Autodesk Inventor part; units mm, degrees
ref_plane "YZ Plane" through (0, 0, 0) normal (1, 0, 0) x (0, 1, 0)
ref_plane "XZ Plane" through (0, 0, 0) normal (0, 1, 0) x (-1, 0, 0)
ref_plane "XY Plane" through (0, 0, 0) normal (0, 0, 1) x (1, 0, 0)
sketch "Sketch1" plane through (0, 0, 0) normal (0, 1, 0) x (-1, 0, 0)
  circle A0 centre (0, 0) radius 1.5
  dimension "d1" = 3
extrude "Extrusion1" add sketch "Sketch1" along normal blind 6
sketch "Sketch2" plane through (0, 6, 0) normal (0, 1, 0) x (1, 0, 0)
  circle A0 centre (0, 0) radius 2.75
  dimension "d4" = 5.5
extrude "Extrusion2" add sketch "Sketch2" along normal blind 3
sketch "Sketch3" plane through (0, 9, 0) normal (0, 1, 0) x (1, 0, 0)
  line L0 (1.5, 0) -> (0.75, -1.299)
  line L1 (0.75, -1.299) -> (-0.75, -1.299)
  line L2 (-0.75, -1.299) -> (-1.5, 0)
  line L3 (-1.5, 0) -> (-0.75, 1.299)
  line L4 (-0.75, 1.299) -> (0.75, 1.299)
  line L5 (0.75, 1.299) -> (1.5, 0)
  point P0 (0, 0)
  point P1 (0, 0)
  dimension "d7" = 1.5
extrude "Extrusion3" cut sketch "Sketch3" against normal blind 2
thread "Thread1"
fillet "Fillet1" radius 0.3 2 edges at (-2.75, 6, 0) (-2.75, 9, 0)
chamfer "Chamfer1" distance 0.05 angle 45 1 edges at (1.5, 0, 0)
chamfer "Chamfer2" distance 0.05 angle 45 1 edges at (1.5, 6, 0)
fillet "Fillet2" radius 0.05 12 edges at (0, 9, -1.299) (1.125, 9, -0.6495) (1.125, 9, 0.6495) (0, 9, 1.299) (-1.125, 9, 0.6495) (-1.125, 9, -0.6495) (0, 7, -1.299) (1.125, 7, -0.6495) (1.125, 7, 0.6495) (-1.125, 7, -0.6495) (-1.125, 7, 0.6495) (0, 7, 1.299)
sketch "Sketch4" plane through (0, 0, 0) normal (0, -1, 0) x (1, 0, 0)
  circle A0 centre (0, 0) radius 1.425
  dimension "d21" = 2.85
extrude "Extrusion4" cut sketch "Sketch4" against normal blind 0.1
chamfer "Chamfer3" distance 0.05 angle 45 1 edges at (-1.425, 0.1, 0)
properties part number "L Bolt M3 x 6 Stainless Steel"
Build history of the part. All positions in model axes, mm. A direction names the side the tool comes from. Round coordinates to 2 decimals unless told otherwise and drop trailing zeros. Write each loop counter-clockwise with the first axis right and the second up, starting at its lowest first coordinate (ties: lowest second). Pieces come first, ordered by that corner, then holes. Notation, with made-up numbers: (-7, -19.75) - (44, -19.75) arc R22 ccw to (44, -1.75) - close; hole circle Ø10 at (82, -15.75). An arc over 180 degrees is marked (long way). Write each question's results on one line, items separated by ' | '. Start each with the question number.
Item 1: Which spindle directions (+Z, -Z, +X, -X, +Y, -Y) get a long thin tool onto all of the face, cutting with end or side? Do faces 1 (the face through (0, 6, 2)), 2 (the face through (0, 8, -1.299)), 3 (the face through (-0.596, 7.483, -2.685)). Say none if no direction does.
Item 2: Saw through at B-B (y = 1.5). Write the cut outline in (x, z), and give its area (3 significant figures).
Item 3: Mould opens along Z. For faces 4 (the face through (0, 7, 0)), 5 (the face through (-1.12, 8.01, 0.66)), 6 (the face through (1.5, 2.96, -0.07)), 7 (the face through (1.1, 9, 1.1)) say: pulls with the +Z half, pulls with the -Z half, needs draft (parallel to the pull), parting line crosses it, or undercut.
Item 4: Wall check: L1, parallel to Y at x = -0.4, z = -0.65; L2, parallel to Z at x = -1.3, y = 2.75; L3, parallel to Y at x = -1.9, z = -0.15. Give the ranges that are in metal, low to high. Write a range as [from, to].
Item 5: Drop flat-ended pins along their axis: P1, Ø2, axis at x = 0, z = 0, coming from the +Y side; P2, Ø0.8, axis at x = 0, z = -0.5, coming from the -Y side; P3, Ø2, axis at x = -0.5, y = 6.5, coming from the +Z side. Give the stop position or say it passes through.
Results are:
1) face 1: -Y | face 2: +Y | face 3: +Y, -Y
2) outline: circle Ø3 at (0, 0) | area: 7.07 mm²
3) face 4: undercut | face 5: undercut | face 6: parting line crosses it | face 7: needs draft
4) L1: y = [0.1, 7] | L2: z = [-0.75, 0.75] | L3: y = [6, 9]
5) P1: stops at y = 7 | P2: stops at y = 0.1 | P3: stops at z = 2.75
